from build123d import *

# Parameters (mm, degrees)
CROQUIS1_R              = 105
SALIENTE_EXTRUIR1_DEPTH = 10
CROQUIS2_R              = 105
CROQUIS3_W              = 280
CROQUIS3_H              = 322
SALIENTE_EXTRUIR2_DEPTH = 8
CROQUIS6_R              = 9.525
CORTAR_EXTRUIR1_DEPTH   = 10


with BuildPart() as part:
    # Croquis1 → Saliente-Extruir1 (new body)
    with BuildSketch(Plane.XY):
        Circle(CROQUIS1_R)
    extrude(amount=SALIENTE_EXTRUIR1_DEPTH)

    # Barrer1: sweep along a curve in space
    with BuildLine() as barrer1_path:
        Line((0, 0, 10), (0, 0, 280))
        ThreePointArc((0, 0, 280), (0, -38.076118446, 371.923881554), (0, -130, 410))
        Line((0, -130, 410), (0, -300, 410))
    # Croquis2 → Barrer1 (sweep)
    with BuildSketch(Plane.XY.offset(10)):
        Circle(CROQUIS2_R)
    sweep(path=barrer1_path.line)

    # Croquis3 → Saliente-Extruir2 (add)
    with BuildSketch(Plane(origin=(0, 0, 0), x_dir=(-1, 0, 0), z_dir=(0, 0, -1))):
        Rectangle(CROQUIS3_W, CROQUIS3_H)
    extrude(amount=-SALIENTE_EXTRUIR2_DEPTH)

    # Croquis6 → Cortar-Extruir1 (cut)
    with BuildSketch(Plane(origin=(0, 0, 0), x_dir=(-1, 0, 0), z_dir=(0, 0, -1))):
        with Locations((0, 131)):
            Circle(CROQUIS6_R)
        with Locations((-110, 61)):
            Circle(CROQUIS6_R)
        with Locations(Location((110, 61, 0), (0, 0, 180))):
            Circle(CROQUIS6_R)
        with Locations((110, -61)):
            Circle(CROQUIS6_R)
        with Locations(Location((-110, -61, 0), (0, 0, 180))):
            Circle(CROQUIS6_R)
        with Locations(Location((0, -131, 0), (0, 0, 180))):
            Circle(CROQUIS6_R)
    extrude(amount=-CORTAR_EXTRUIR1_DEPTH, mode=Mode.SUBTRACT)


solid = part.part
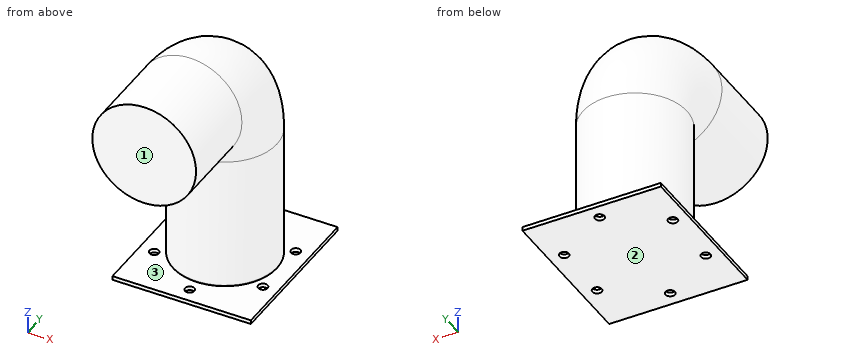
Geometry: final body of the model. Coordinates: model frame, mm. Face numbers are marked on the shaded views. Coordinates: 2 decimals unless noted, no trailing zeros. Loops run counter-clockwise (first coordinate to the right, second up) from the corner with the lowest first, then second, coordinate; pieces in that order, holes last. Notation, with made-up numbers: M 24.5,24.5 L 55.5,24.5 A26 ccw 55.5,52.5 Z; hole C 21,32.5 d5. An arc over 180 degrees is marked long. One line per item, written item: value. Start each with the question number.
1) Cut plane B-B (x = 0). Return loops of the section in (y, z) (3 decimals), then the cut area to 3 significant figures.
2) Pin query (flat end, axial travel): P1, Ø6, axis at x = 70, z = 312.5, coming from the -Y side; P2, Ø5, axis at y = 75.5, z = 160, coming from the -X side; P3, Ø12, axis at x = 91.5, y = 57.5, coming from the -Z side; P4, Ø1.5, axis at x = -44.5, z = 285.5, coming from the -Y side. Return the tip coordinate at first contact, or that it passes through.
3) Material intervals for L1, parallel to Y at x = 0, z = 5 (3 decimals); L2, parallel to Y at x = 110, z = 5 (3 decimals); L3, parallel to X at y = -3.5, z = 239, sorted ascending. Write a range as from..to.
4) Cut plane A-A (y = 131). Return loops of the section in (x, z) (3 decimals), then the cut area to 3 significant figures.
5) Draft query along Z for the marked faces 1, 2 and 3. Return one class per face: released by +Z, released by -Z, zero draft, split by the parting line, or undercut.
6) Cut plane D-D (x = -54.5). Return loops of the section in (y, z).
7) Cut plane C-C (y = -254). Return loops of the section in (x, z), then the cut area to 3 significant figures.
Evaluation:
1. outline: M -300,305 L -130,305 A25 cw -105,280 L -105,8 L -121.475,8 L -121.475,0 L 121.475,0 L 121.475,8 L 105,8 L 105,280 A235 ccw -130,515 L -300,515 Z; M -161,0 L -140.525,0 L -140.525,8 L -161,8 Z; M 140.525,0 L 161,0 L 161,8 L 140.525,8 Z
1. area: 138,000 mm^2
2. P1: y = -94.1
2. P2: x = -75.47
2. P3: z = 0
2. P4: y = -95.91
3. L1: -161..-140.525, -121.475..121.475, 140.525..161
3. L2: -161..-70.525, -51.475..51.475, 70.525..161
3. L3: -104.94..104.94
4. outline: M -140,0 L -9.525,0 L -9.525,8 L -140,8 Z; M 9.525,0 L 140,0 L 140,8 L 9.525,8 Z
4. area: 2,090 mm^2
5. face 1: zero draft
5. face 2: released by -Z
5. face 3: undercut
6. outline: M -300,320.25 L -130,320.25 A40.25 cw -89.75,280 L -89.75,8 L -161,8 L -161,0 L 161,0 L 161,8 L 89.75,8 L 89.75,280 A219.75 ccw -130,499.75 L -300,499.75 Z
7. outline: C 0,410 d210
7. area: 34,600 mm^2
